from build123d import *

# Parameters (mm, degrees)
SKETCH1_R                                      = 4
BOSS_EXTRUDE1_DEPTH                            = 19.05
SKETCH2_R                                      = 11.1125
BOSS_EXTRUDE2_DEPTH                            = 3.175
CUT_EXTRUDE2_START                             = -1.5875
SKETCH10_R                                     = 11.1125
CUT_EXTRUDE2_DEPTH                             = 1.5875
CSK_FOR_M3_FLAT_HEAD_MACHINE_SCREW1_AT_2_COUNT = 2
CSK_FOR_M3_FLAT_HEAD_MACHINE_SCREW1_AT_2_PITCH = 11.225320151
CSK_FOR_M3_FLAT_HEAD_MACHINE_SCREW1_AT_3_COUNT = 2
CSK_FOR_M3_FLAT_HEAD_MACHINE_SCREW1_AT_3_PITCH = 11.225320151
CSK_FOR_M3_FLAT_HEAD_MACHINE_SCREW1_AT_4_COUNT = 2
CSK_FOR_M3_FLAT_HEAD_MACHINE_SCREW1_AT_4_PITCH = 15.875


with BuildPart() as part:
    # Sketch1 → Boss-Extrude1 (new body)
    with BuildSketch(Plane(origin=(0, 0, 0), x_dir=(1, 0, 0), z_dir=(0, 1, 0))):
        with Locations(Location((0, 0, 0), (0, 0, 270))):
            Circle(SKETCH1_R)
    extrude(amount=-BOSS_EXTRUDE1_DEPTH)

    # Sketch2 → Boss-Extrude2 (add)
    with BuildSketch(Plane(origin=(0, 0, 0), x_dir=(1, 0, 0), z_dir=(0, 1, 0))):
        with Locations(Location((0, 0, 0), (0, 0, 270))):
            Circle(SKETCH2_R)
    extrude(amount=BOSS_EXTRUDE2_DEPTH)

    # Sketch10 → Cut-Extrude2 (cut)
    with BuildSketch(Plane(origin=(0, 3.175, 0), x_dir=(1, 0, 0), z_dir=(0, 1, 0)).offset(CUT_EXTRUDE2_START)):
        with Locations(Location((0, 0, 0), (0, 0, 270))):
            Circle(SKETCH10_R)
    extrude(amount=CUT_EXTRUDE2_DEPTH, mode=Mode.SUBTRACT)

    # Sketch6 → CSK for M3 Flat Head Machine Screw1 (revolve, cut)
    with BuildSketch(Plane(origin=(7.9375, 1.5875, 0), x_dir=(0, 0, 1), z_dir=(1, 0, 0))):
        Polygon((0, 0), (0, 1.5875), (1.7, 1.5875), (1.7, 1.45), (3.15, 0), align=None)
    csk_for_m3_flat_head_machine_screw1 = revolve(axis=Axis((7.9375, 7.9375, 0), (0, -1, 0)), mode=Mode.SUBTRACT)

    # CSK for M3 Flat Head Machine Screw1 at 2: CSK for M3 Flat Head Machine Screw1 ×2
    with Locations(*[Vector(-0.7071067811865476, 0, -0.7071067811865476) * (i * CSK_FOR_M3_FLAT_HEAD_MACHINE_SCREW1_AT_2_PITCH) for i in range(1, CSK_FOR_M3_FLAT_HEAD_MACHINE_SCREW1_AT_2_COUNT)]):
        add(csk_for_m3_flat_head_machine_screw1, mode=Mode.SUBTRACT)

    # CSK for M3 Flat Head Machine Screw1 at 3: CSK for M3 Flat Head Machine Screw1 ×2
    with Locations(*[Vector(-0.7071067811865476, 0, 0.7071067811865476) * (i * CSK_FOR_M3_FLAT_HEAD_MACHINE_SCREW1_AT_3_PITCH) for i in range(1, CSK_FOR_M3_FLAT_HEAD_MACHINE_SCREW1_AT_3_COUNT)]):
        add(csk_for_m3_flat_head_machine_screw1, mode=Mode.SUBTRACT)

    # CSK for M3 Flat Head Machine Screw1 at 4: CSK for M3 Flat Head Machine Screw1 ×2
    with Locations(*[(-i * CSK_FOR_M3_FLAT_HEAD_MACHINE_SCREW1_AT_4_PITCH, 0, 0) for i in range(1, CSK_FOR_M3_FLAT_HEAD_MACHINE_SCREW1_AT_4_COUNT)]):
        add(csk_for_m3_flat_head_machine_screw1, mode=Mode.SUBTRACT)


solid = part.part
Source: CAD feature listing. Evaluate the final solid. Frame: model axes, mm. A direction names the side the tool comes from. Round coordinates to 2 decimals unless told otherwise and drop trailing zeros. Loops run counter-clockwise (first coordinate to the right, second up) from the corner with the lowest first, then second, coordinate; pieces in that order, holes last.
Q1. First-contact query: P1, Ø4, axis at x = 0, z = 7.94, coming from the +Y side; P2, Ø5, axis at y = -12.5, z = 3, coming from the -X side; P3, Ø12, axis at x = 0, y = -13, coming from the +Z side. Flat tips, straight axial feed; report the tip coordinate or a pass-through.
Q2. Section C-C, the plane y = -9.75. Return loops of the section in (x, z).
Q3. Section A-A, the plane x = 0. State how many separate pieces and enclosed holes the cut face has, plus the area to 3 significant figures.
Q4. Access query for faces 1 (the face through (-5, 0, 0)), 2 (the face through (9.37, 0.783, 5.974)). Directions: +Z, -Z, +X, -X, +Y, -Y. A direction counts if a zero-diameter tool reaches every point of the face in a straight line with its end or side. Return the directions, or none.
Q5. Ray query, line 1 (Z direction, x = -0.5, y = 0.25); line 2 (Y direction, x = 2.25, z = 5); line 3 (X direction, y = -14, z = 0). Return the intervals inside material, ascending.
Solutions:
1. P1: stops at y = 0.44
1. P2: stops at x = -3.97
1. P3: stops at z = 4
2. outline: circle Ø8 at (0, 0)
3. separate pieces: 3
3. enclosed holes: 0
3. area: 173 mm2
4. face 1: -Y
4. face 2: +Y, -Y
5. line 1: z = -11.1 to -9.68, -6.2 to 6.2, 9.68 to 11.1
5. line 2: y = 0 to 1.59
5. line 3: x = -4 to 4
